Could you check a few things on this model? Use its own coordinates, in mm. Coordinates: 2 decimals unless noted, no trailing zeros. Write each loop counter-clockwise with the first axis right and the second up, starting at its lowest first coordinate (ties: lowest second). Pieces come first, ordered by that corner, then holes.
Item 1: I want a section at A-A on z = 6.25. State how many separate pieces and enclosed holes the cut face has, then the cut area to 3 significant figures.
Item 2: For P1, Ø3, axis at x = 0, y = 70, coming from the +Z side; P2, Ø4, axis at x = -50, y = 49, coming from the +Z side; P3, Ø1.5, axis at x = 20, z = 6, coming from the +Y side; P4, Ø1.5, axis at y = -60, z = 4.5, coming from the +X side, each with a flat end and sliding along its axis, tell me the tip position at first contact or that it passes through.
Item 3: I want a section at B-B on x = 12. Please give me the cut outline in (y, z), then the cut area to 3 significant figures.
Item 4: I want a section at D-D on x = -50. Please give me the cut outline in (y, z).
Item 5: If I drill on probe 1 along Y at (x, z) = (-1, 0.5); probe 2 along Y at (x, z) = (49.49, 6.55); probe 3 along Y at (x, z) = (18.2, 5.85), over which ranges is the centre line in solid material (lowest first)?
Item 6: I want a section at C-C on y = 25.5. Please give me the cut outline in (x, z), then the cut area to 3 significant figures.
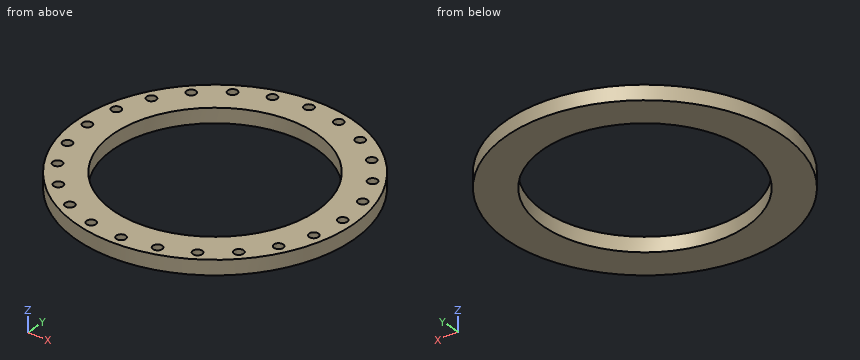
from build123d import *

# Parameters (mm, degrees)
CYLINDER001002001001_R           = 2.6
CYLINDER001002001001_DEPTH       = 20
CYLINDER001002001001001_R        = 2.6
CYLINDER001002001001001_DEPTH    = 20
CYLINDER001002001001001001_R     = 2.6
CYLINDER001002001001001001_DEPTH = 26
CYLINDER001002_R                 = 2.6
CYLINDER001002_DEPTH             = 20
CYLINDER001002001_R              = 2.6
CYLINDER001002001_DEPTH          = 20
CYLINDER001_R                    = 2.6
CYLINDER001_DEPTH                = 20
CYLINDER001001_R                 = 2.6
CYLINDER001001_DEPTH             = 20
CYLINDER002_R                    = 56
CYLINDER002_DEPTH                = 10
CYLINDER_R                       = 76
CYLINDER_DEPTH                   = 8


with BuildPart() as pole003:
    # Cylinder001002001001 → Cylinder001002001001 (new body)
    with BuildSketch(Plane(origin=(60.62, 35, 3), x_dir=(1, 0, 0), z_dir=(0, 0, 1))):
        Circle(CYLINDER001002001001_R)
    extrude(amount=CYLINDER001002001001_DEPTH)


with BuildPart() as pole004:
    # Cylinder001002001001001 → Cylinder001002001001001 (new body)
    with BuildSketch(Plane(origin=(49.49, 49.49, 3), x_dir=(1, 0, 0), z_dir=(0, 0, 1))):
        Circle(CYLINDER001002001001001_R)
    extrude(amount=CYLINDER001002001001001_DEPTH)


with BuildPart() as pole005:
    # Cylinder001002001001001001 → Cylinder001002001001001001 (new body)
    with BuildSketch(Plane(origin=(35, 60.62, 3), x_dir=(1, 0, 0), z_dir=(0, 0, 1))):
        Circle(CYLINDER001002001001001001_R)
    extrude(amount=CYLINDER001002001001001001_DEPTH)


with BuildPart() as cylinder001002:
    # Cylinder001002 → Cylinder001002 (new body)
    with BuildSketch(Plane(origin=(18.2, 67.55, 3), x_dir=(1, 0, 0), z_dir=(0, 0, 1))):
        Circle(CYLINDER001002_R)
    extrude(amount=CYLINDER001002_DEPTH)


with BuildPart() as pole2:
    # Cylinder001002001 → Cylinder001002001 (new body)
    with BuildSketch(Plane(origin=(67.55, 18.2, 3), x_dir=(1, 0, 0), z_dir=(0, 0, 1))):
        Circle(CYLINDER001002001_R)
    extrude(amount=CYLINDER001002001_DEPTH)


with BuildPart() as fusion:
    # Fusion base: copy of pole2
    add(pole2.part)

    # Fusion: union pole003, pole004, pole005, Cylinder001002
    add(pole003.part)
    add(pole004.part)
    add(pole005.part)
    add(cylinder001002.part)


with BuildPart() as part_mirroring:
    # Part__Mirroring: instance of Fusion
    add(fusion.part.mirror(Plane(origin=(0, 0, 0), x_dir=(1, 0, 0), z_dir=(0, 1, 0))))


with BuildPart() as pole1:
    # Cylinder001 → Cylinder001 (new body)
    with BuildSketch(Plane(origin=(70, 0, 3), x_dir=(1, 0, 0), z_dir=(0, 0, 1))):
        Circle(CYLINDER001_R)
    extrude(amount=CYLINDER001_DEPTH)


with BuildPart() as part_mirroring001:
    # Part__Mirroring001: instance of Fusion
    add(fusion.part.mirror(Plane(origin=(3e-06, 42.766762, 16), x_dir=(0, -1, 0), z_dir=(1, 0, 0))))


with BuildPart() as part_mirroring003:
    # Part__Mirroring003: instance of pole1
    add(pole1.part.mirror(Plane(origin=(0, 0, 0), x_dir=(0, -1, 0), z_dir=(1, 0, 0))))


with BuildPart() as part_mirroring002:
    # Part__Mirroring002: instance of Part__Mirroring
    add(part_mirroring.part.mirror(Plane(origin=(0, 0, 0), x_dir=(0, -1, 0), z_dir=(1, 0, 0))))


with BuildPart() as cylinder001001:
    # Cylinder001001 → Cylinder001001 (new body)
    with BuildSketch(Plane(origin=(0, 70, 3), x_dir=(1, 0, 0), z_dir=(0, 0, 1))):
        Circle(CYLINDER001001_R)
    extrude(amount=CYLINDER001001_DEPTH)


with BuildPart() as part_mirroring004:
    # Part__Mirroring004: instance of Cylinder001001
    add(cylinder001001.part.mirror(Plane(origin=(0, 0, 0), x_dir=(1, 0, 0), z_dir=(0, 1, 0))))


with BuildPart() as fusion001:
    # Fusion001 base: copy of Cylinder001001
    add(cylinder001001.part)

    # Fusion001: union Part__Mirroring, pole1, Fusion, pole2, pole003, pole004, pole005, Cylinder001002, Part__Mirroring001, Part__Mirroring003, Part__Mirroring002, Part__Mirroring004
    add(part_mirroring.part)
    add(pole1.part)
    add(fusion.part)
    add(pole2.part)
    add(pole003.part)
    add(pole004.part)
    add(pole005.part)
    add(cylinder001002.part)
    add(part_mirroring001.part)
    add(part_mirroring003.part)
    add(part_mirroring002.part)
    add(part_mirroring004.part)


with BuildPart() as cylinder002:
    # Cylinder002 → Cylinder002 (new body)
    with BuildSketch(Plane.XY):
        Circle(CYLINDER002_R)
    extrude(amount=CYLINDER002_DEPTH)


with BuildPart() as cut001:
    # Cylinder → Cylinder (new body)
    with BuildSketch(Plane.XY):
        Circle(CYLINDER_R)
    extrude(amount=CYLINDER_DEPTH)

    # Cut: cut Cylinder002
    add(cylinder002.part, mode=Mode.SUBTRACT)

    # Cut001: cut Fusion001
    add(fusion001.part, mode=Mode.SUBTRACT)


solid = cut001.part
Response values:
1. separate pieces: 1
1. enclosed holes: 25
1. area: 7,780 mm2
2. P1: stops at z = 3
2. P2: stops at z = 8
2. P3: stops at y = 73.52
2. P4: stops at x = 47.6
3. outline: (-75.05, 0) - (-54.7, 0) - (-54.7, 8) - (-75.05, 8) - close; (54.7, 0) - (75.05, 0) - (75.05, 8) - (54.7, 8) - close
3. area: 326 mm2
4. outline: (-57.24, 0) - (-25.22, 0) - (-25.22, 8) - (-46.94, 8) - (-46.94, 3) - (-52.04, 3) - (-52.04, 8) - (-57.24, 8) - close; (25.22, 0) - (57.24, 0) - (57.24, 8) - (52.04, 8) - (52.04, 3) - (46.94, 3) - (46.94, 8) - (25.22, 8) - close
5. probe 1: y = -75.99 to -55.99, 55.99 to 75.99
5. probe 2: y = -57.68 to -52.09, -46.89 to -26.21, 26.21 to 46.89, 52.09 to 57.68
5. probe 3: y = -73.79 to -70.15, -64.95 to -52.96, 52.96 to 64.95, 70.15 to 73.79
6. outline: (-71.59, 0) - (-49.86, 0) - (-49.86, 8) - (-71.59, 8) - close; (49.86, 0) - (71.59, 0) - (71.59, 8) - (49.86, 8) - close
6. area: 348 mm2
